Could you check a few things on this drawing? It's one solid part, dimensions in mm from its lowest x, y, z. Coordinates: 2 decimals unless noted, no trailing zeros. Order: outer loops, then holes, each group sorted by start corner. A loop starts at its lowest first (then second) coordinate and runs counter-clockwise, first axis right, second up. Notation, with made-up numbers: (26, -4.75) -> (51, -4.75) arc R28 cw to (51, 28.25) -> close; hole circle Ø9 at (31, -34). An arc over 180 degrees is marked (long way). Use a Markdown table: item, result. Add a question column.
1. We'd pull the mould along Z, two halves only. Please class the marked faces 1, 2 and 3: pulls with the +Z half, pulls with the -Z half, needs draft (parallel to the pull), parting line crosses it, or undercut.
2. If I drill on line 1 along X through (y, z) = (23, 371.5); line 2 along Z through (x, y) = (528.5, 8); line 3 along Y through (x, z) = (723, 581), over which ranges is the centre line in solid material (lowest first)? Write a range as from..to.
3. Suppose I cut it at A-A, the plane z = 359.5. List the corners of the cut face in (x, y) for me, then the cut area to 3 significant figures.
4. Suppose I cut it at D-D, the plane y = 63.5. List the corners of the cut face in (x, z) for me, then the cut area to 3 significant figures.
5. For pin 1 Ø2 at (x, y) = (503.5, 83) entering from +Z; pin 2 Ø3 at (x, z) = (939, 289.5) entering from -Y; pin 3 Ø12 at (x, y) = (255, 58.5) entering from +Z, each with a flat end and sliding along its axis, tell me the tip position at first contact or that it passes through.
6. Suppose I cut it at B-B, the plane y = 12.5. List the corners of the cut face in (x, z) for me, then the cut area to 3 significant figures.
7. Suppose I cut it at C-C, the plane x = 165. List the corners of the cut face in (y, z) for me.
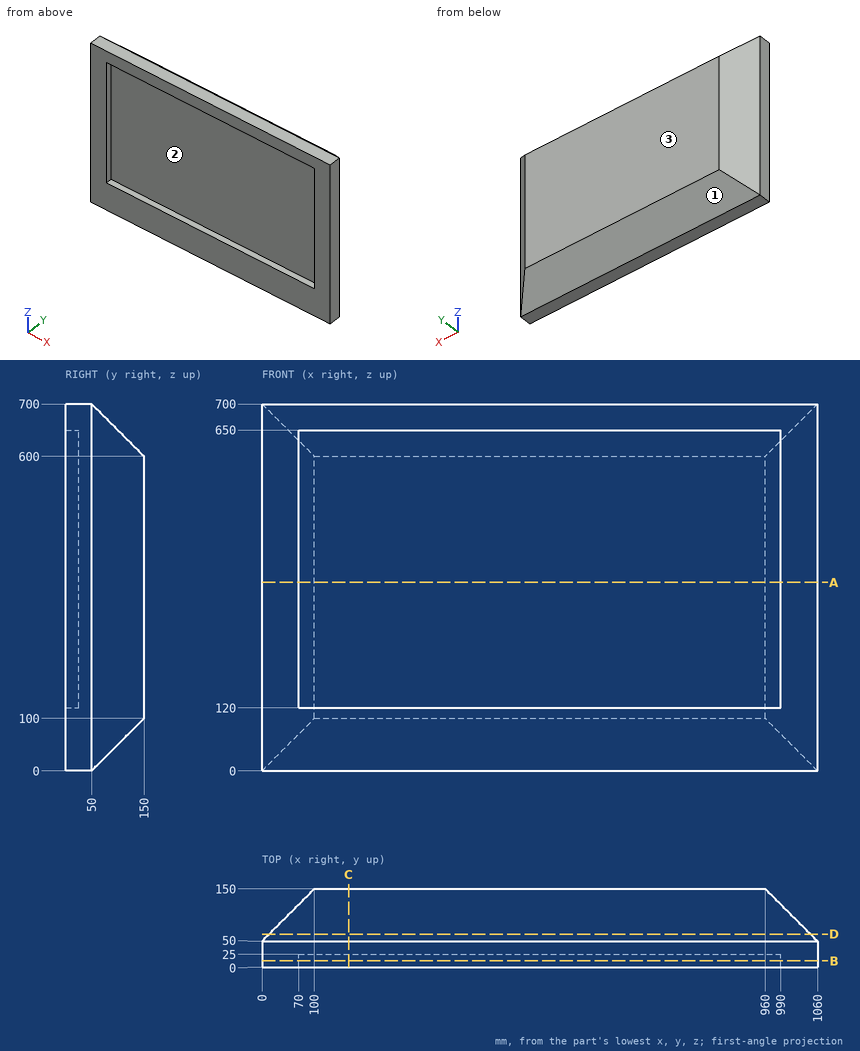
Worked out:
| question | item | result |
|---|---|---|
| 1 | face 1 | pulls with the -Z half |
| 1 | face 2 | undercut |
| 1 | face 3 | needs draft |
| 2 | line 1 | x = 0..70, 990..1060 |
| 2 | line 2 | z = 0..120, 650..700 |
| 2 | line 3 | y = 25..150 |
| 3 | outline | (0, 0) -> (70, 0) -> (70, 25) -> (990, 25) -> (990, 0) -> (1060, 0) -> (1060, 50) -> (960, 150) -> (100, 150) -> (0, 50) -> close |
| 3 | area | 126,000 mm² |
| 4 | outline | (13.5, 13.5) -> (1046.5, 13.5) -> (1046.5, 686.5) -> (13.5, 686.5) -> close |
| 4 | area | 695,000 mm² |
| 5 | pin 1 | stops at z = 668 |
| 5 | pin 2 | stops at y = 25 |
| 5 | pin 3 | stops at z = 697.5 |
| 6 | outline | (0, 0) -> (1060, 0) -> (1060, 700) -> (0, 700) -> close; hole (70, 120) -> (990, 120) -> (990, 650) -> (70, 650) -> close |
| 6 | area | 254,000 mm² |
| 7 | outline | (0, 0) -> (50, 0) -> (150, 100) -> (150, 600) -> (50, 700) -> (0, 700) -> (0, 650) -> (25, 650) -> (25, 120) -> (0, 120) -> close |
